```python
from build123d import *

# Parameters (mm, degrees)
F0_W     = 76.2
F0_H     = 114.3
F1_DEPTH = 9.525
F3_D     = 4.2
F6_D     = 3.3
F6_DEPTH = 12
F6_TIP   = 0.9914200214


# Not quite as in the source:
# - a pattern or mirror of a feature is missing from the dataset's text; its kind, count and spacing are read off the source's solid
# - a feature names something its author has since deleted; it is built from what else it names


with BuildPart() as f1:
    # F0 (on Top) → F1 (new body)
    with BuildSketch(Plane.XY):
        Rectangle(F0_W, F0_H)
    extrude(amount=F1_DEPTH)

    # F3 (through all)
    with Locations(Plane.XY.offset(9.525)):
        with Locations((-31.75, 52.3875), (31.75, 52.3875), (31.75, -52.3875), (-31.75, -52.3875)):
            Hole(F3_D / 2)

    # F6
    with Locations(Plane.XY.offset(9.525)):
        with Locations((-25.9, -19.15), (25.9, -19.15)):
            f6 = Hole(F6_D / 2, depth=F6_DEPTH)
            with Locations((0, 0, -(F6_DEPTH + F6_TIP / 2))):  # 118° drill point
                Cone(0, F6_D / 2, F6_TIP, mode=Mode.SUBTRACT)

    # F6_copies: F6 across plane
    add(f6.mirror(Plane.ZX), mode=Mode.SUBTRACT)


solid = f1.part
```
Design review of the part built by this model. Coordinates are the model's own, in mm. Coordinates: 2 decimals unless noted, no trailing zeros. Write each loop counter-clockwise with the first axis right and the second up, starting at its lowest first coordinate (ties: lowest second). Pieces come first, ordered by that corner, then holes.
1) Insertion check: pin 1 (2.5 mm diameter, centred on x = 25.9, y = 19.15, fed in from +Z). The pin has a flat end and moves straight along its axis. Give the tip position at first contact, or say it passes through.
2) Add section B-B (y = -19.15). Write out the cut boundary in (x, z) (3 decimals), plus the area to 3 significant figures.
3) Add section A-A (x = -25.9). Write out the cut boundary in (y, z) (3 decimals), plus the area to 3 significant figures.
4) To check wall thickness, follow L1, parallel to Y at x = 25.9, z = 7; L2, parallel to Y at x = 31.75, z = 2.25; L3, parallel to X at y = -19, z = 5. State the ranges of each line that lie inside material, in increasing order.
5) Mouldability with a two-part tool opening along X and no side actions: class faces 1 (the flat face through (-38.1, -1, 5)), 2 (the cylindrical face through (-26.661, 20.614, 4.696)), 3 (the flat face through (-1, 1, 0)) as +X half, -X half, draft (parallel to the pull), parting line (faces both ways), or undercut.
Check result:
1. pin 1: passes through
2. outline: (-38.1, 0) - (-27.55, 0) - (-27.55, 9.525) - (-38.1, 9.525) - close; (-24.25, 0) - (24.25, 0) - (24.25, 9.525) - (-24.25, 9.525) - close; (27.55, 0) - (38.1, 0) - (38.1, 9.525) - (27.55, 9.525) - close
2. area: 663 mm2
3. outline: (-57.15, 0) - (-20.8, 0) - (-20.8, 9.525) - (-57.15, 9.525) - close; (-17.5, 0) - (17.5, 0) - (17.5, 9.525) - (-17.5, 9.525) - close; (20.8, 0) - (57.15, 0) - (57.15, 9.525) - (20.8, 9.525) - close
3. area: 1,030 mm2
4. L1: y = -57.15 to -20.8, -17.5 to 17.5, 20.8 to 57.15
4. L2: y = -57.15 to -54.49, -50.29 to 50.29, 54.49 to 57.15
4. L3: x = -38.1 to -27.54, -24.26 to 24.26, 27.54 to 38.1
5. face 1: -X half
5. face 2: undercut
5. face 3: draft
